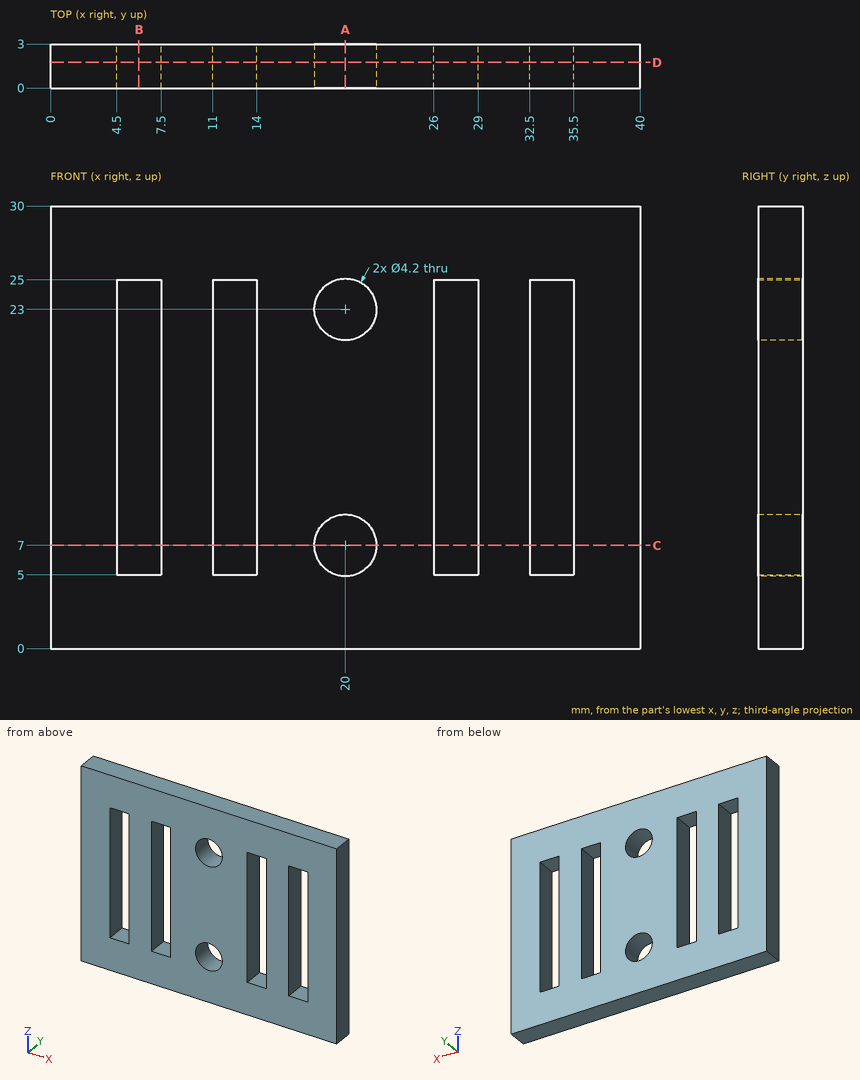
Geometry check sheet. Reference: drawing and pictorial views, mm from the part's lowest x, y, z. Give positions to 0.01 mm unless a question says otherwise; leave off trailing zeros. Write each loop counter-clockwise with the first axis right and the second up, starting at its lowest first coordinate (ties: lowest second). Pieces come first, ordered by that corner, then holes. Notation, with made-up numbers: (-7, -28) -> (28, -28) arc R24 cw to (28, -8) -> close; hole circle Ø1 at (-9.75, -10.5). An arc over 180 degrees is marked (long way). One line per item, written item: value. Start each with the question number.
Item 1: Material ranges on probe 1 along X at (y, z) = (0.5, 20.75); probe 2 along X at (y, z) = (0.7, 23); probe 3 along Z at (x, y) = (13, 1.25), recorded low to high. Write a range as from..to.
Item 2: Section check D-D on y = 1.75. Record the cut outline in (x, z), then the cut area to 3 significant figures.
Item 3: Section check C-C on z = 7. Record the cut outline in (x, y), then the cut area to 3 significant figures.
Item 4: Section check B-B on x = 6. Record the cut outline in (y, z).
Item 5: Section check A-A on x = 20. Record the cut outline in (y, z).
Results list:
1. probe 1: 0..4.5, 7.5..11, 14..26, 29..32.5, 35.5..40
1. probe 2: 0..4.5, 7.5..11, 14..17.9, 22.1..26, 29..32.5, 35.5..40
1. probe 3: 0..5, 25..30
2. outline: (0, 0) -> (40, 0) -> (40, 30) -> (0, 30) -> close; hole (4.5, 5) -> (7.5, 5) -> (7.5, 25) -> (4.5, 25) -> close; hole (11, 5) -> (14, 5) -> (14, 25) -> (11, 25) -> close; hole circle Ø4.2 at (20, 7); hole circle Ø4.2 at (20, 23); hole (26, 5) -> (29, 5) -> (29, 25) -> (26, 25) -> close; hole (32.5, 5) -> (35.5, 5) -> (35.5, 25) -> (32.5, 25) -> close
2. area: 932 mm²
3. outline: (0, 0) -> (4.5, 0) -> (4.5, 3) -> (0, 3) -> close; (7.5, 0) -> (11, 0) -> (11, 3) -> (7.5, 3) -> close; (14, 0) -> (17.9, 0) -> (17.9, 3) -> (14, 3) -> close; (22.1, 0) -> (26, 0) -> (26, 3) -> (22.1, 3) -> close; (29, 0) -> (32.5, 0) -> (32.5, 3) -> (29, 3) -> close; (35.5, 0) -> (40, 0) -> (40, 3) -> (35.5, 3) -> close
3. area: 71.4 mm²
4. outline: (0, 0) -> (3, 0) -> (3, 5) -> (0, 5) -> close; (0, 25) -> (3, 25) -> (3, 30) -> (0, 30) -> close
5. outline: (0, 0) -> (3, 0) -> (3, 4.9) -> (0, 4.9) -> close; (0, 9.1) -> (3, 9.1) -> (3, 20.9) -> (0, 20.9) -> close; (0, 25.1) -> (3, 25.1) -> (3, 30) -> (0, 30) -> close
